Can you work these out from the model? Positions are in its coordinate system, mm. Face numbers are marked on the shaded views. A direction names the side the tool comes from. Coordinates: 2 decimals unless noted, no trailing zeros. Loops run counter-clockwise (first coordinate to the right, second up) from the corner with the lowest first, then second, coordinate; pieces in that order, holes last. Notation, with made-up numbers: (62, -5.5) - (100, -5.5) arc R22 cw to (100, 3.5) - close; hole circle Ø10 at (35.25, -25). An arc over 180 degrees is marked (long way). Put each result on its own line as item: value. Start each with the question number.
from build123d import *

# Parameters (mm, degrees)
ESQUISSE1_W             = 7
ESQUISSE1_H             = 30
BOSS_EXTRU_1_DEPTH      = 35
ESQUISSE2_R             = 8
ENL_V_MAT_EXTRU_1_DEPTH = 28
ESQUISSE4_R             = 1.8
ENL_V_MAT_EXTRU_2_DEPTH = 10
ESQUISSE4_3_R           = 13.4
ESQUISSE4_3_R_2         = 1.8
ESQUISSE4_3_R_3         = 7
ENL_V_MAT_EXTRU_3_DEPTH = 4
ESQUISSE4_4_R           = 7
ENL_V_MAT_EXTRU_4_DEPTH = 10
ESQUISSE4_11_W          = 18
ESQUISSE4_11_H          = 3
BOSS_EXTRU_2_DEPTH      = 55
ESQUISSE8_W             = 8
ESQUISSE8_H             = 8
ESQUISSE8_R             = 2.3
BOSS_EXTRU_3_DEPTH      = 6
ESQUISSE10_W            = 16
ESQUISSE10_H            = 12
BOSS_EXTRU_4_DEPTH      = 7
ESQUISSE9_R             = 1.8
ENL_V_MAT_EXTRU_5_DEPTH = 10
ESQUISSE11_R            = 1.6
ENL_V_MAT_EXTRU_6_DEPTH = 10
ESQUISSE12_R            = 2.5
ENL_V_MAT_EXTRU_7_DEPTH = 1
ESQUISSE15_R            = 8
ENL_V_MAT_EXTRU_8_DEPTH = 10
BOSS_EXTRU_5_DEPTH      = 15


with BuildPart() as part:
    # Esquisse1 → Boss.-Extru.1 (new body)
    with BuildSketch(Plane(origin=(0, 0, 0), x_dir=(1, 0, 0), z_dir=(0, 1, 0))):
        with Locations((-13.5, 91)):
            Rectangle(ESQUISSE1_W, ESQUISSE1_H)
        Polygon((-17, 0), (0, 0), (17, 0), (17, 50), (10, 50), (10, 6), (-10, 6), (-10, 76), (-17, 76), align=None)
    extrude(amount=BOSS_EXTRU_1_DEPTH)

    # Esquisse2 → Enl_v. mat.-Extru.1 (cut)
    with BuildSketch(Plane(origin=(17, 0, 0), x_dir=(0, 0, -1), z_dir=(1, 0, 0))):
        with Locations((30, 18)):
            Circle(ESQUISSE2_R)
    extrude(amount=-ENL_V_MAT_EXTRU_1_DEPTH, mode=Mode.SUBTRACT)

    # Esquisse4 → Enl_v. mat.-Extru.2 (cut)
    with BuildSketch(Plane.ZY.offset(17)):
        with Locations((-98, 18)):
            Circle(ESQUISSE4_R)
        with Locations((-88, 28)):
            Circle(ESQUISSE4_R)
        with Locations((-88, 8)):
            Circle(ESQUISSE4_R)
        with Locations((-78, 18)):
            Circle(ESQUISSE4_R)
    extrude(amount=-ENL_V_MAT_EXTRU_2_DEPTH, mode=Mode.SUBTRACT)

    # Esquisse4_3 → Enl_v. mat.-Extru.3 (cut)
    with BuildSketch(Plane.ZY.offset(17)):
        with Locations((-88, 18)):
            Circle(ESQUISSE4_3_R)
        with Locations((-98, 18)):
            Circle(ESQUISSE4_3_R_2, mode=Mode.SUBTRACT)
        with Locations((-88, 28)):
            Circle(ESQUISSE4_3_R_2, mode=Mode.SUBTRACT)
        with Locations((-78, 18)):
            Circle(ESQUISSE4_3_R_2, mode=Mode.SUBTRACT)
        with Locations((-88, 8)):
            Circle(ESQUISSE4_3_R_2, mode=Mode.SUBTRACT)
        with Locations((-88, 18)):
            Circle(ESQUISSE4_3_R_3, mode=Mode.SUBTRACT)
    extrude(amount=-ENL_V_MAT_EXTRU_3_DEPTH, mode=Mode.SUBTRACT)

    # Esquisse4_4 → Enl_v. mat.-Extru.4 (cut)
    with BuildSketch(Plane.ZY.offset(17)):
        with Locations((-88, 18)):
            Circle(ESQUISSE4_4_R)
    extrude(amount=-ENL_V_MAT_EXTRU_4_DEPTH, mode=Mode.SUBTRACT)

    # Esquisse4_11 → Boss.-Extru.2 (add)
    with BuildSketch(Plane.ZY.offset(17)):
        Polygon((-106, 0), (-97, 0), (-97, 3), (-97, 8), (-106, 8), align=None)
        Polygon((-70, 0), (-70, 8), (-79, 8), (-79, 3), (-79, 0), align=None)
        with Locations((-88, 1.5)):
            Rectangle(ESQUISSE4_11_W, ESQUISSE4_11_H)
    extrude(amount=BOSS_EXTRU_2_DEPTH)

    # Esquisse8 → Boss.-Extru.3 (add)
    # profile 1 of 5: a face of its own
    with BuildSketch(Plane.XZ):
        with Locations((13, 4)):
            Rectangle(ESQUISSE8_W, ESQUISSE8_H)
        with Locations(Location((13, 4, 0), (0, 0, 270))):
            Circle(ESQUISSE8_R, mode=Mode.SUBTRACT)
    # profile 2 of 5: a face of its own
    with BuildSketch(Plane.XZ):
        with Locations((-13, 4)):
            Rectangle(ESQUISSE8_W, ESQUISSE8_H)
        with Locations(Location((-13, 4, 0), (0, 0, 270))):
            Circle(ESQUISSE8_R, mode=Mode.SUBTRACT)
    # profile 3 of 5: a face of its own
    with BuildSketch(Plane.XZ):
        with Locations((-68, -110)):
            Rectangle(ESQUISSE8_W, ESQUISSE8_H)
        with Locations(Location((-68, -110, 0), (0, 0, 270))):
            Circle(ESQUISSE8_R, mode=Mode.SUBTRACT)
    # profile 4 of 5: a face of its own
    with BuildSketch(Plane.XZ):
        with Locations((-68, -66)):
            Rectangle(ESQUISSE8_W, ESQUISSE8_H)
        with Locations(Location((-68, -66, 0), (0, 0, 270))):
            Circle(ESQUISSE8_R, mode=Mode.SUBTRACT)
    # profile 5 of 5: a face of its own
    with BuildSketch(Plane.XZ):
        with Locations((-14, -110)):
            Rectangle(ESQUISSE8_W, ESQUISSE8_H)
        with Locations(Location((-14, -110, 0), (0, 0, 270))):
            Circle(ESQUISSE8_R, mode=Mode.SUBTRACT)
    extrude(amount=-BOSS_EXTRU_3_DEPTH)

    # Esquisse10 → Boss.-Extru.4 (add)
    with BuildSketch(Plane.ZY.offset(17)):
        with Locations((-55, 41)):
            Rectangle(ESQUISSE10_W, ESQUISSE10_H)
    extrude(amount=-BOSS_EXTRU_4_DEPTH)

    # Esquisse9 → Enl_v. mat.-Extru.5 (cut)
    with BuildSketch(Plane.ZY.offset(17)):
        with Locations((-55, 28)):
            Circle(ESQUISSE9_R)
        with BuildLine():
            ThreePointArc((-56.8, 28), (-55, 29.8), (-53.2, 28))
            Line((-53.2, 28), (-53.2, 42))
            ThreePointArc((-53.2, 42), (-55, 40.2), (-56.8, 42))
            Line((-56.8, 42), (-56.8, 28))
        make_face()
        with Locations((-55, 42)):
            Circle(ESQUISSE9_R)
    extrude(amount=-ENL_V_MAT_EXTRU_5_DEPTH, mode=Mode.SUBTRACT)

    # Esquisse11 → Enl_v. mat.-Extru.6 (cut)
    with BuildSketch(Plane(origin=(0, 35, 0), x_dir=(1, 0, 0), z_dir=(0, 1, 0))):
        with Locations(Location((-13.5, 30, 0), (0, 0, 270))):
            Circle(ESQUISSE11_R)
        with Locations(Location((13.5, 30, 0), (0, 0, 270))):
            Circle(ESQUISSE11_R)
    extrude(amount=-ENL_V_MAT_EXTRU_6_DEPTH, mode=Mode.SUBTRACT)

    # Esquisse12 → Enl_v. mat.-Extru.7 (cut)
    with BuildSketch(Plane(origin=(-10, 0, 0), x_dir=(0, 0, -1), z_dir=(1, 0, 0))):
        with Locations((88, 28)):
            Circle(ESQUISSE12_R)
        with Locations((98, 18)):
            Circle(ESQUISSE12_R)
        with Locations((88, 8)):
            Circle(ESQUISSE12_R)
        with Locations((78, 18)):
            Circle(ESQUISSE12_R)
    extrude(amount=-ENL_V_MAT_EXTRU_7_DEPTH, mode=Mode.SUBTRACT)

    # Esquisse15 → Enl_v. mat.-Extru.8 (cut)
    with BuildSketch(Plane(origin=(-11, 0, 0), x_dir=(0, 0, -1), z_dir=(1, 0, 0))):
        with Locations(Location((30, 18, 0), (0, 0, 180))):
            Circle(ESQUISSE15_R)
    extrude(amount=-ENL_V_MAT_EXTRU_8_DEPTH, mode=Mode.SUBTRACT)

    # Esquisse16 → Boss.-Extru.5 (add)
    with BuildSketch(Plane.ZY.offset(72)):
        Polygon((-106, 8), (-106, 0), (-70, 0), (-70, 8), (-79, 8), (-79, 3), (-97, 3), (-97, 8), align=None)
    extrude(amount=BOSS_EXTRU_5_DEPTH)


solid = part.part
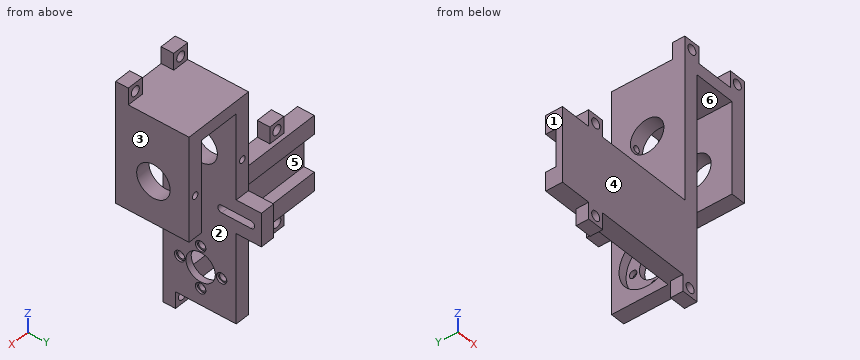
Q1. We'd pull the mould along X, two halves only. Please class the marked faces 1, 2 and 3: released by +X, released by -X, zero draft, split by the parting line, or undercut.
Q2. I want a section at B-B on z = 4. List the corners of the cut face in (x, y) for me, and give its area (3 significant figures).
Q3. I want a section at D-D on x = -1. List the corners of the cut face in (y, z) for me.
Q4. On a 3-axis mill with a long thin cutter (end or side, diameter ignored), from which of +Z, -Z, +X, -X, +Y, -Y can I reach the whole of each face in a straight line? I mean the marked faces 4, 5 and 6. Say none if no direction works.
Q5. Will these pins go through, and if not, where does the flat tip stop? pin 1 (1 mm diameter, centred on y = 27.5, z = -80.5, fed in from -X); pin 2 (5 mm diameter, centred on y = 17, z = -11, fed in from -X); pin 3 (4 mm diameter, centred on x = -13, z = -111.5, fed in from +Y); pin 4 (11 mm diameter, centred on y = 18, z = -88, fed in from -X) (3 decimals).
Q6. I want a section at C-C on x = -45.5. List the corners of the cut face in (y, z) for me, and give its area (3 significant figures).
Q7. Please list where these lines run through material, in increasing order: line 1 along X through (y, z) = (4, 4); line 2 along Y through (x, z) = (-12, -88); line 3 along Y through (x, z) = (-10.4, -88). Write a range as [from, to].
Calculated:
1. face 1: released by -X
1. face 2: undercut
1. face 3: released by +X
2. outline: (-17, 0) - (-15.3, 0) - (-15.3, 6) - (-17, 6) - close; (-10.7, 0) - (-9, 0) - (-9, 6) - (-10.7, 6) - close; (9, 0) - (10.7, 0) - (10.7, 6) - (9, 6) - close; (15.3, 0) - (17, 0) - (17, 6) - (15.3, 6) - close
2. area: 40.8 mm2
3. outline: (0, -6) - (35, -6) - (35, 0) - (0, 0) - close
4. face 4: +Z, -Z, +X, -X, -Y
4. face 5: -X, +Y
4. face 6: -Z, +Y, -Y
5. pin 1: x = -13
5. pin 2: x = -17
5. pin 3: y = 6
5. pin 4: through
6. outline: (0, -106) - (8, -106) - (8, -97) - (3, -97) - (3, -79) - (8, -79) - (8, -70) - (0, -70) - close
6. area: 198 mm2
7. line 1: [-17, -15.3], [-10.7, -9], [9, 10.7], [15.3, 17]
7. line 2: [0, 6.2], [9.8, 11], [25, 26.2], [29.8, 35]
7. line 3: [0, 5.5], [10.5, 11], [25, 25.5], [30.5, 35]
